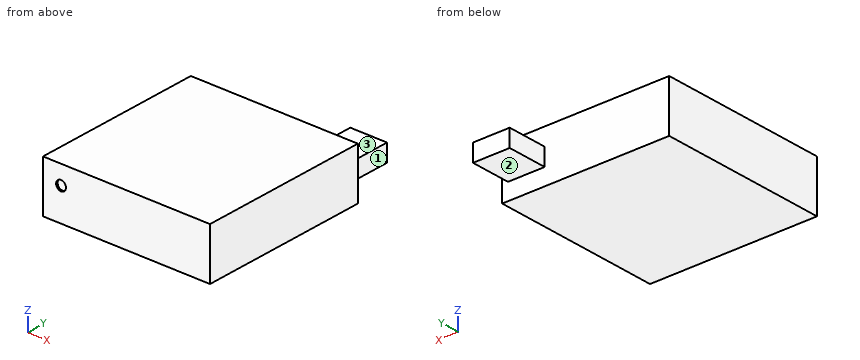
from build123d import *

# Parameters (mm, degrees)
F0_W     = 195
F0_H     = 200
F1_DEPTH = 60
F2_W     = 42.843923
F2_H     = 20.3234
F3_DEPTH = 47.3
F4_R     = 5.719599
F5_DEPTH = 2


with BuildPart() as f1:
    # F0 (on Top) → F1 (new body)
    with BuildSketch(Plane.XY):
        Rectangle(F0_W, F0_H)
    extrude(amount=F1_DEPTH)

    # F2 (on face) → F3 (join)
    with BuildSketch(Plane(origin=(0, 100, 0), x_dir=(-1, 0, 0), z_dir=(0, 1, 0))):
        with Locations((-69.346733, 29.588042)):
            Rectangle(F2_W, F2_H)
    extrude(amount=F3_DEPTH)

    # F4 (on face) → F5 (cut)
    with BuildSketch(Plane.XZ.offset(100)):
        with Locations((-76.43842, 38.019974)):
            Circle(F4_R)
    extrude(amount=-F5_DEPTH, mode=Mode.SUBTRACT)


solid = f1.part
Can you work these out from the model? Positions are in its coordinate system, mm. Face numbers are marked on the shaded views. A direction names the side the tool comes from. Give positions to 0.01 mm unless a question says otherwise; leave off trailing zeros. Loops run counter-clockwise (first coordinate to the right, second up) from the corner with the lowest first, then second, coordinate; pieces in that order, holes last. Notation, with made-up numbers: (16.25, 83) -> (48.25, 83) arc R25 cw to (48.25, 103) -> close; hole circle Ø7 at (-11.75, 83). An arc over 180 degrees is marked (long way). Return JSON: item names as keys, results as strings.
Q1. I need wall thicknesses on probe 1 along Y at (x, z) = (40, 26.5); probe 2 along Z at (x, y) = (84, 113); probe 3 along X at (y, z) = (109.5, 23.5). Which ranges of each line are inside material? Lowest first, please.
Checks:
{"probe 1": "y = -100 to 100", "probe 2": "z = 19.43 to 39.75", "probe 3": "x = 47.92 to 90.77"}
Q2. On a 3-axis mill with a long thin cutter (end or side, diameter ignored), from which of +Z, -Z, +X, -X, +Y, -Y can I reach the whole of each face in a straight line? I mean the marked faces 1, 2 and 3. Say none if no direction works.
Checks:
{"face 1": "+Z, -Z, +X, +Y", "face 2": "-Z, +X, -X, +Y", "face 3": "+Z, +X, -X, +Y"}
Q3. I want a section at B-B, the plane x = 34.5. List the corners of the cut face in (y, z) for me, then the cut area to 3 significant figures.
Checks:
{"outline": "(-100, 0) -> (100, 0) -> (100, 60) -> (-100, 60) -> close", "area": "12,000 mm2"}
Q4. I want a section at A-A, the plane z = 13. List the corners of the cut face in (x, y) for me.
Checks:
{"outline": "(-97.5, -100) -> (97.5, -100) -> (97.5, 100) -> (-97.5, 100) -> close"}
Q5. For pin 1 Ø13 at (x, y) = (77, 130.5) entering from -Z; pin 2 Ø3 at (y, z) = (111, 28) entering from -X; pin 3 Ø12 at (x, z) = (-76, 43.5) entering from +Y, each with a flat end and sliding along its axis, tell me the tip position at first contact or that it passes through.
Checks:
{"pin 1": "stops at z = 19.43", "pin 2": "stops at x = 47.92", "pin 3": "stops at y = 100"}
